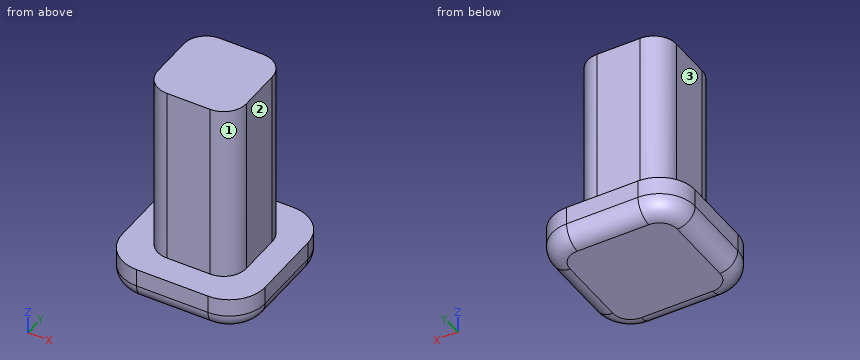
Autodesk Fusion 360 part; units mm, degrees
sketch "Base" plane through (0, 0, 0) normal (0, 0, 1) x (1, 0, 0)
  line L0 (3, 0) -> (9, 0)
  line L1 (12, 3) -> (12, 9)
  line L2 (9, 12) -> (3, 12)
  line L3 (0, 9) -> (0, 3)
  arc A0 (3, 12) -> (0, 9) centre (3, 9) ccw
  arc A1 (12, 9) -> (9, 12) centre (9, 9) ccw
  arc A2 (9, 0) -> (12, 3) centre (9, 3) ccw
  arc A3 (0, 3) -> (3, 0) centre (3, 3) ccw
  point P0 (12, 0)
  point P1 (0, 12)
  dimension "d1" = 12
  dimension "d2" = 12
  dimension "d3" = 3
sketch "Sketch2" plane through (0, 0, 3) normal (0, 0, 1) x (-1, 0, 0)
  arc A0 (0, -3) -> (-3, 0) centre (-3, -3) ccw
  arc A1 (-3, -12) -> (0, -9) centre (-3, -9) ccw
  line L0 (-4.18, -2.28) -> (-7.82, -2.28)
  line L1 (-9.72, -4.18) -> (-9.72, -7.82)
  line L2 (-7.82, -9.72) -> (-4.18, -9.72)
  line L3 (-2.28, -7.82) -> (-2.28, -4.18)
  arc A2 (-4.18, -9.72) -> (-2.28, -7.82) centre (-4.18, -7.82) ccw
  arc A3 (-9.72, -7.82) -> (-7.82, -9.72) centre (-7.82, -7.82) ccw
  arc A4 (-7.82, -2.28) -> (-9.72, -4.18) centre (-7.82, -4.18) ccw
  arc A5 (-2.28, -4.18) -> (-4.18, -2.28) centre (-4.18, -4.18) ccw
  point P0 (-2.28, -2.28)
  point P1 (-9.72, -2.28)
  point P2 (-2.28, -9.72)
  dimension "d18" = 7.44
  dimension "d19" = 7.44
  dimension "d20" = 1.9
extrude "Extrude3" add sketch "Base" along normal blind 3
extrude "Extrude4" add sketch "Sketch2" along normal blind 15.143
fillet "Fillet2" radius 1.5 8 edges at (12, 6, 0) (11.1213, 11.1213, 0) (6, 12, 0) (0.8787, 11.1213, 0) (0, 6, 0) (0.8787, 0.8787, 0) (6, 0, 0) (11.1213, 0.8787, 0)
The model under review builds one solid part; all positions refer to its coordinate system, in mm. Face numbers are marked on the shaded views. A direction names the side the tool comes from. Round coordinates to 2 decimals unless told otherwise and drop trailing zeros. Write each loop counter-clockwise with the first axis right and the second up, starting at its lowest first coordinate (ties: lowest second). Pieces come first, ordered by that corner, then holes. Notation, with made-up numbers: (6.5, 14) - (52.5, 14) arc R36 ccw to (52.5, 51) - close; hole circle Ø5 at (29, 28). An arc over 180 degrees is marked (long way). Answer as CSV lines item,"result". Start each with the question number.
(1) For the marked faces 1, 2 and 3, list the 3-axis set-ups (+Z, -Z, +X, -X, +Y, -Y) from which the entire face can be reached by the end or side of a thin tool; tool diameter is ignored.
(2) For pin 1 Ø3 at (y, z) = (5, 13.5) entering from +X; pin 2 Ø1.8 at (x, z) = (6.5, 7.5) entering from -Y; pin 3 Ø1.1 at (y, z) = (5.5, 12) entering from -X, all flat-tipped, find the tip position at first contact; note any pin that passes through.
(3) We need section B-B on z = 2.5. State the section outline as (x, y) points, plus the area to 3 significant figures.
(4) We need section A-A on x = 6.75. State the section outline as (y, z) points, plus the area to 3 significant figures.
(5) To check wall thickness, follow line 1 (X direction, y = 7, z = 15.5); line 2 (Z direction, x = 1.5, y = 5.5). State the ranges of each line that lie inside material, in increasing order.
Worked answers:
1,face 1,"+Z, +X, -Y"
1,face 2,"+Z, +X, +Y, -Y"
1,face 3,"+Z, -X, +Y, -Y"
2,pin 1,"x = 9.72"
2,pin 2,"y = 2.28"
2,pin 3,"x = 2.28"
3,outline,"(0, 3) arc R3 ccw to (3, 0) - (9, 0) arc R3 ccw to (12, 3) - (12, 9) arc R3 ccw to (9, 12) - (3, 12) arc R3 ccw to (0, 9) - close"
3,area,"136 mm²"
4,outline,"(0, 1.5) arc R1.5 ccw to (1.5, 0) - (10.5, 0) arc R1.5 ccw to (12, 1.5) - (12, 3) - (9.72, 3) - (9.72, 18.14) - (2.28, 18.14) - (2.28, 3) - (0, 3) - close"
4,area,"148 mm²"
5,line 1,"2.28 to 9.72"
5,line 2,"0 to 3"
